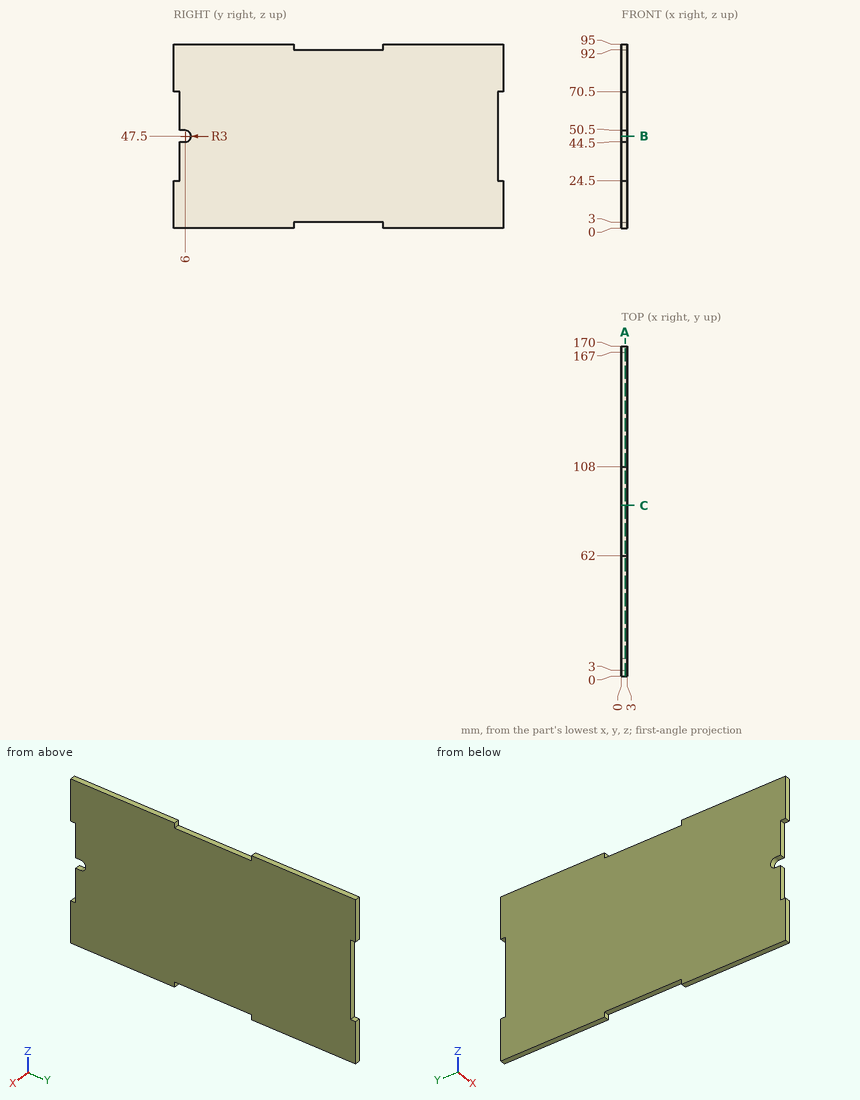
Geometry check sheet. Reference: drawing and pictorial views, mm from the part's lowest x, y, z. Coordinates: 2 decimals unless noted, no trailing zeros. Order: outer loops, then holes, each group sorted by start corner. A loop starts at its lowest first (then second) coordinate and runs counter-clockwise, first axis right, second up.
Item 1: Depth check by flat-ended pin: pin 1 (3 mm diameter, centred on y = 100, z = 53.5, fed in from -X); pin 2 (0.9 mm diameter, centred on x = 1, y = 89.5, fed in from -Z); pin 3 (1.5 mm diameter, centred on x = 1, z = 55, fed in from +Y). Enter the tip coordinate at first touch or a pass-through.
Filled in:
pin 1: stops at x = 0
pin 2: stops at z = 3
pin 3: stops at y = 167
Item 2: Section check B-B, the plane z = 47.5. Enter the section's corners in (x, y).
Filled in:
outline: (0, 9) - (3, 9) - (3, 167) - (0, 167) - close
Item 3: Section check A-A, the plane x = 1.9. Enter the section's corners in (y, z).
Filled in:
outline: (0, 0) - (62, 0) - (62, 3) - (108, 3) - (108, 0) - (170, 0) - (170, 24.5) - (167, 24.5) - (167, 70.5) - (170, 70.5) - (170, 95) - (108, 95) - (108, 92) - (62, 92) - (62, 95) - (0, 95) - (0, 70.5) - (3, 70.5) - (3, 50.5) - (6, 50.5) arc R3 cw to (6, 44.5) - (3, 44.5) - (3, 24.5) - (0, 24.5) - close
Item 4: Section check C-C, the plane y = 88. Enter the section's corners in (x, z).
Filled in:
outline: (0, 3) - (3, 3) - (3, 92) - (0, 92) - close
Item 5: Material ranges on L1, parallel to Z at x = 1.65, y = 64; L2, parallel to Y at x = 1.55, z = 66.5; L3, parallel to Y at x = 0.95, z = 45.5, recorded low to high.
Filled in:
L1: z = 3 to 92
L2: y = 3 to 167
L3: y = 8.24 to 167
